Verification items for the finished model (mm, model axes). Face numbers are marked on the shaded views. A direction names the side the tool comes from. Give positions to 0.01 mm unless a question says otherwise; leave off trailing zeros. Order: outer loops, then holes, each group sorted by start corner. A loop starts at its lowest first (then second) coordinate and runs counter-clockwise, first axis right, second up. Notation, with made-up numbers: (81, -13.5) - (124, -13.5) arc R16 cw to (124, -6.5) - close; hole circle Ø2 at (72.5, 58.5). An arc over 180 degrees is marked (long way). Answer as a JSON object with one key per item and string values.
Autodesk Inventor part; units mm, degrees
ref_plane "Plano de trabajo1" through (0, 0, 31.375) normal (0, 0, 1) x (1, 0, 0)
ref_plane "YZ Plane" through (0, 0, 0) normal (1, 0, 0) x (0, 1, 0)
ref_plane "XZ Plane" through (0, 0, 0) normal (0, 1, 0) x (-1, 0, 0)
sketch "Boceto1" plane through (0, 0, 0) normal (0, 0, 1) x (1, 0, 0)
  circle A0 centre (0, 0) radius 3
  dimension "d0" = 6
extrude "Extrusión1" add sketch "Boceto1" along normal blind 26
sketch "Boceto2" plane through (0, 0, 26) normal (0, 0, 1) x (1, 0, 0)
  line L0 (6, 0) -> (3, -5.1962)
  line L1 (3, -5.1962) -> (-3, -5.1962)
  line L2 (-3, -5.1962) -> (-6, 0)
  line L3 (-6, 0) -> (-3, 5.1962)
  line L4 (-3, 5.1962) -> (3, 5.1962)
  line L5 (3, 5.1962) -> (6, 0)
  point P0 (0, 0)
  point P1 (0, 0)
  point P2 (0, 5.1962)
  dimension "d3" = 6
extrude "Extrusión2" add sketch "Boceto2" along normal blind 10.75
ref_plane "Plano de trabajo1" through (0, 0, 31.375) normal (0, 0, 1) x (1, 0, 0)
mirror "Simetría1" about plane through (0, 0, 31.375) normal (0, 0, 1) of "Extrusión1"
properties part number "wheel_shock_pin"
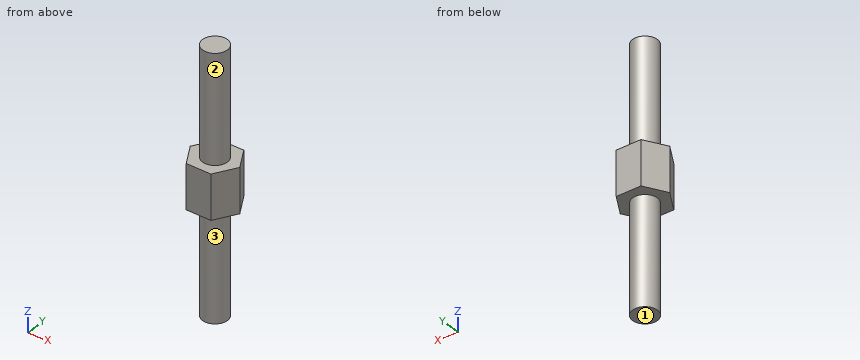
(1) Section check D-D (x = -5). Record the cut outline in (y, z), then the cut area to 3 significant figures.
Computed values:
{"outline": "(-1.73, 26) - (1.73, 26) - (1.73, 36.75) - (-1.73, 36.75) - close", "area": "37.2 mm²"}
(2) Section check B-B (y = 1.5). Record the cut outline in (x, z), then the cut area to 3 significant figures.
Computed values:
{"outline": "(-5.13, 26) - (-2.6, 26) - (-2.6, 0) - (2.6, 0) - (2.6, 26) - (5.13, 26) - (5.13, 36.75) - (2.6, 36.75) - (2.6, 62.75) - (-2.6, 62.75) - (-2.6, 36.75) - (-5.13, 36.75) - close", "area": "381 mm²"}
(3) Material ranges on line 1 along Z through (x, y) = (-5, 1.25); line 2 along X through (y, z) = (-2, 55); line 3 along X through (y, z) = (-2.25, 18), recorded low to high. Write a range as [from, to].
Computed values:
{"line 1": "z = [26, 36.75]", "line 2": "x = [-2.24, 2.24]", "line 3": "x = [-1.98, 1.98]"}
(4) Access from +Z, -Z, +X, -X, +Y, -Y to the whole of each face (thin tool, end or side, straight path). Record for the marked faces 1, 2 and 3.
Computed values:
{"face 1": "-Z, +X, -X, +Y, -Y", "face 2": "+Z", "face 3": "-Z"}
(5) Gauge pin test, flat ends, axial feed: pin 1 Ø2 at (y, z) = (-1, 14) entering from -X; pin 2 Ø2 at (x, z) = (1, 49) entering from +Y; pin 3 Ø5 at (x, y) = (-1, -1.5) entering from -Z; pin 4 Ø1.5 at (x, z) = (1.5, 53.5) entering from -Y. Record the tip position at first contact, or that the pin passes through.
Computed values:
{"pin 1": "stops at x = -3", "pin 2": "stops at y = 3", "pin 3": "stops at z = 0", "pin 4": "stops at y = -2.9"}
(6) Section check A-A (x = 0). Record the cut outline in (y, z), then the cut area to 3 significant figures.
Computed values:
{"outline": "(-5.2, 26) - (-3, 26) - (-3, 0) - (3, 0) - (3, 26) - (5.2, 26) - (5.2, 36.75) - (3, 36.75) - (3, 62.75) - (-3, 62.75) - (-3, 36.75) - (-5.2, 36.75) - close", "area": "424 mm²"}
(7) Section check C-C (z = 14.5). Record the cut outline in (x, y).
Computed values:
{"outline": "circle Ø6 at (0, 0)"}
